```python
from build123d import *

# Parameters (mm, degrees)
F1_R      = 20
F2_DEPTH  = 1.2
F3_R      = 20
F4_DEPTH  = 1.2
F6_R      = 20
F6_R_2    = 18.8
F7_DEPTH  = 50
F9_R      = 20
F11_R     = 4.1
F13_DEPTH = 12
F15_R     = 3
F16_DEPTH = 25
F14_R     = 18.8


# Not quite as in the source:
# - after a boolean that leaves OpenCascade's solid faulty, fix() repairs it


with BuildPart() as f2:
    # F1 (on Top) → F2 (new body)
    with BuildSketch(Plane.XY):
        Circle(F1_R)
        with BuildLine():
            Line((-18.7904230926, -0.6), (-0.6, -0.6))
            Line((-0.6, -0.6), (-0.6, -18.7904230926))
            ThreePointArc((-0.6, -18.7904230926), (-13.2936074863, -13.2936074863), (-18.7904230926, -0.6))
        make_face(mode=Mode.SUBTRACT)
        with BuildLine():
            Line((0.6, -18.7904230926), (0.6, -0.6))
            Line((0.6, -0.6), (18.7904230926, -0.6))
            ThreePointArc((18.7904230926, -0.6), (13.2936074863, -13.2936074863), (0.6, -18.7904230926))
        make_face(mode=Mode.SUBTRACT)
        with BuildLine():
            Line((-0.6, 18.7904230926), (-0.6, 0.6))
            Line((-0.6, 0.6), (-18.7904230926, 0.6))
            ThreePointArc((-18.7904230926, 0.6), (-13.2936074863, 13.2936074863), (-0.6, 18.7904230926))
        make_face(mode=Mode.SUBTRACT)
        with BuildLine():
            Line((18.7904230926, 0.6), (0.6, 0.6))
            Line((0.6, 0.6), (0.6, 18.7904230926))
            ThreePointArc((0.6, 18.7904230926), (13.2936074863, 13.2936074863), (18.7904230926, 0.6))
        make_face(mode=Mode.SUBTRACT)
    extrude(amount=F2_DEPTH)

    # F3 (on Top) → F4 (join)
    with BuildSketch(Plane.XY):
        Circle(F3_R)
    extrude(amount=-F4_DEPTH)

    # F6 (on offset) → F7 (join)
    with BuildSketch(Plane.XY.offset(1.2)):
        Circle(F6_R)
        Circle(F6_R_2, mode=Mode.SUBTRACT)
    extrude(amount=F7_DEPTH)

    add(f2.part.fix(), mode=Mode.REPLACE)

    # F9 (on offset) → F12 section 0
    with BuildSketch(Plane.XY.offset(51.2)):
        Circle(F9_R)
    # F11 (on offset) → F12 section 1
    with BuildSketch(Plane.XY.offset(71.2)):
        Circle(F11_R)
    loft()

    # F13 (add): a face of the model
    f13_faces = [f2.faces().sort_by_distance(p)[0] for p in [
        (0, 0, 71.2),
    ]]
    extrude(f13_faces, amount=F13_DEPTH)

    # F15 (on offset) → F16 (cut)
    with BuildSketch(Plane.XY.offset(71.2)):
        Circle(F15_R)
    extrude(amount=F16_DEPTH, mode=Mode.SUBTRACT)

    # F14 (on offset) → F17 section 0
    with BuildSketch(Plane.XY.offset(51.2)):
        Circle(F14_R)
    # F15 (on offset) → F17 section 1
    with BuildSketch(Plane.XY.offset(71.2)):
        Circle(F15_R)
    loft(mode=Mode.SUBTRACT)


solid = f2.part
```
Can you work these out from the model? Positions are in its coordinate system, mm. A direction names the side the tool comes from. Round coordinates to 2 decimals unless told otherwise and drop trailing zeros. Loops run counter-clockwise (first coordinate to the right, second up) from the corner with the lowest first, then second, coordinate; pieces in that order, holes last. Notation, with made-up numbers: (19, -15) -> (71, -15) arc R30 cw to (71, 20) -> close; hole circle Ø3 at (-30, 63.5). An arc over 180 degrees is marked (long way). Answer in a Markdown table with one row per item.
Item 1: On a 3-axis mill with a long thin cutter (end or side, diameter ignored), from which of +Z, -Z, +X, -X, +Y, -Y can I reach the whole of each face in a straight line? I mean faces 4 (the conical face through (6.33, 1.99, 68.01)), 5 (the flat face through (-8, 8, 0)). Say none if no direction works.
Answer block:
| item | result |
|---|---|
| face 4 | +Z |
| face 5 | none |
Item 2: Will these pins go through, and if not, where does the flat tip stop? P1, Ø1, axis at y = 6.5, z = 0.5, coming from the -X side; P2, Ø9, axis at x = 7.5, y = -13, coming from the +Z side; P3, Ø1, axis at y = -10.5, z = 44.5, coming from the +X side.
Answer block:
| item | result |
|---|---|
| P1 | x = -19.08 |
| P2 | z = 63.14 |
| P3 | x = 17.32 |
Item 3: If I drill on probe 1 along Y at (x, z) = (0, 21); probe 2 along Y at (x, z) = (0, 79); probe 3 along X at (y, z) = (3.5, 46.5), over which ranges is the centre line in solid material (lowest first)?
Answer block:
| item | result |
|---|---|
| probe 1 | -20 to -18.8, 18.8 to 20 |
| probe 2 | -4.1 to -3, 3 to 4.1 |
| probe 3 | -19.69 to -18.47, 18.47 to 19.69 |
Item 4: Suppose I cut it at A-A, the plane z = 9. List the corners of the cut face in (x, y) for me.
Answer block:
| item | result |
|---|---|
| outline | circle Ø40 at (0, 0); hole circle Ø37.6 at (0, 0) |
Item 5: We'd pull the mould along X, two halves only. Please class faces 1 (the cylindrical face through (-3, 0, 77)), 2 (the flat face through (0, 0, -1.2)), 3 (the cylindrical face through (-0.534, 4.065, 77.116)): released by +X, released by -X, zero draft, split by the parting line, or undercut.
Answer block:
| item | result |
|---|---|
| face 1 | undercut |
| face 2 | zero draft |
| face 3 | split by the parting line |
Item 6: Suppose I cut it at B-B, the plane z = 77. List the corners of the cut face in (x, y) for me, plus the area to 3 significant figures.
Answer block:
| item | result |
|---|---|
| outline | circle Ø8.2 at (0, 0); hole circle Ø6 at (0, 0) |
| area | 24.5 mm² |
